from build123d import *

# Parameters (mm, degrees)
F1_DEPTH = 1175
F2_R     = 3
F3_DEPTH = 18
F4_R     = 5
F5_DEPTH = 7


with BuildPart() as f1:
    # F0 (on Right) → F1 (new body)
    with BuildSketch(Plane.YZ):
        with BuildLine():
            Line((-26.041336, 5), (-26.041336, 0))
            Line((-26.041336, 0), (-6.041336, 0))
            Line((-6.041336, 0), (-6.041336, 5))
            ThreePointArc((-6.041336, 5), (-9.041336, 8), (-6.041336, 11))
            Line((-6.041336, 11), (-6.041336, 15))
            ThreePointArc((-6.041336, 15), (-8.162657, 15.87868), (-9.041336, 18))
            Line((-9.041336, 18), (-23.041336, 18))
            ThreePointArc((-23.041336, 18), (-23.920016, 15.87868), (-26.041336, 15))
            Line((-26.041336, 15), (-26.041336, 11))
            ThreePointArc((-26.041336, 11), (-23.041336, 8), (-26.041336, 5))
        make_face()
    extrude(amount=F1_DEPTH)

    # F2 (on face) → F3 (cut)
    with BuildSketch(Plane.XY.offset(18)):
        with Locations((17.5, -16.041336)):
            Circle(F2_R)
        with Locations((77.5, -16.041336)):
            Circle(F2_R)
        with Locations((137.5, -16.041336)):
            Circle(F2_R)
        with Locations((197.5, -16.041336)):
            Circle(F2_R)
        with Locations((257.5, -16.041336)):
            Circle(F2_R)
        with Locations((317.5, -16.041336)):
            Circle(F2_R)
        with Locations((377.5, -16.041336)):
            Circle(F2_R)
        with Locations((437.5, -16.041336)):
            Circle(F2_R)
        with Locations((497.5, -16.041336)):
            Circle(F2_R)
        with Locations((557.5, -16.041336)):
            Circle(F2_R)
        with Locations((617.5, -16.041336)):
            Circle(F2_R)
        with Locations((677.5, -16.041336)):
            Circle(F2_R)
        with Locations((737.5, -16.041336)):
            Circle(F2_R)
        with Locations((797.5, -16.041336)):
            Circle(F2_R)
        with Locations((857.5, -16.041336)):
            Circle(F2_R)
        with Locations((917.5, -16.041336)):
            Circle(F2_R)
        with Locations((977.5, -16.041336)):
            Circle(F2_R)
        with Locations((1037.5, -16.041336)):
            Circle(F2_R)
        with Locations((1097.5, -16.041336)):
            Circle(F2_R)
    extrude(amount=-F3_DEPTH, mode=Mode.SUBTRACT)

    # F4 (on face) → F5 (cut)
    with BuildSketch(Plane.XY.offset(18)):
        with Locations((17.5, -16.041336)):
            Circle(F4_R)
        with Locations((77.5, -16.041336)):
            Circle(F4_R)
        with Locations((137.5, -16.041336)):
            Circle(F4_R)
        with Locations((197.5, -16.041336)):
            Circle(F4_R)
        with Locations((257.5, -16.041336)):
            Circle(F4_R)
        with Locations((317.5, -16.041336)):
            Circle(F4_R)
        with Locations((377.5, -16.041336)):
            Circle(F4_R)
        with Locations((437.5, -16.041336)):
            Circle(F4_R)
        with Locations((497.5, -16.041336)):
            Circle(F4_R)
        with Locations((557.5, -16.041336)):
            Circle(F4_R)
        with Locations((617.5, -16.041336)):
            Circle(F4_R)
        with Locations((677.5, -16.041336)):
            Circle(F4_R)
        with Locations((737.5, -16.041336)):
            Circle(F4_R)
        with Locations((797.5, -16.041336)):
            Circle(F4_R)
        with Locations((857.5, -16.041336)):
            Circle(F4_R)
        with Locations((917.5, -16.041336)):
            Circle(F4_R)
        with Locations((977.5, -16.041336)):
            Circle(F4_R)
        with Locations((1037.5, -16.041336)):
            Circle(F4_R)
        with Locations((1097.5, -16.041336)):
            Circle(F4_R)
    extrude(amount=-F5_DEPTH, mode=Mode.SUBTRACT)


solid = f1.part
Could you check a few things on this model? Use its own coordinates, in mm. Give positions to 0.01 mm unless a question says otherwise; leave off trailing zeros. Order: outer loops, then holes, each group sorted by start corner. A loop starts at its lowest first (then second) coordinate and runs counter-clockwise, first axis right, second up.
Item 1: I'm going to push flat-ended pins straight in: pin 1 (5 mm diameter, centred on x = 619.5, y = -16.5, fed in from +Z); pin 2 (5.5 mm diameter, centred on x = 137.5, y = -16.04, fed in from -Z); pin 3 (4 mm diameter, centred on x = 884.5, z = 8.5, fed in from -Y). Where does each tip first touch, or does it pass through?
Item 2: I need wall thicknesses on line 1 (Y direction, x = 737.5, z = 14.5); line 2 (Y direction, x = 377.5, z = 4.75); line 3 (Y direction, x = 337, z = 17.25). Which ranges of each line are inside material? Lowest first, please.
Item 3: If we section it at B-B, the plane z = 8: Count the separate pieces of the cut face and the enclosed holes in it, plus the area to 3 significant figures.
Item 4: If we section it at A-A, the plane x = 395: Write out the boundary of the cut face in (y, z), plus the area to 3 significant figures.
Values:
1. pin 1: stops at z = 11
1. pin 2: passes through
1. pin 3: stops at y = -24.38
2. line 1: y = -26.04 to -21.04, -11.04 to -6.04
2. line 2: y = -26.04 to -19.04, -13.04 to -6.04
2. line 3: y = -23.14 to -8.95
3. separate pieces: 1
3. enclosed holes: 19
3. area: 15,900 mm2
4. outline: (-26.04, 0) - (-6.04, 0) - (-6.04, 5) arc R3 cw to (-6.04, 11) - (-6.04, 15) arc R3 cw to (-9.04, 18) - (-23.04, 18) arc R3 cw to (-26.04, 15) - (-26.04, 11) arc R3 cw to (-26.04, 5) - close
4. area: 318 mm2
